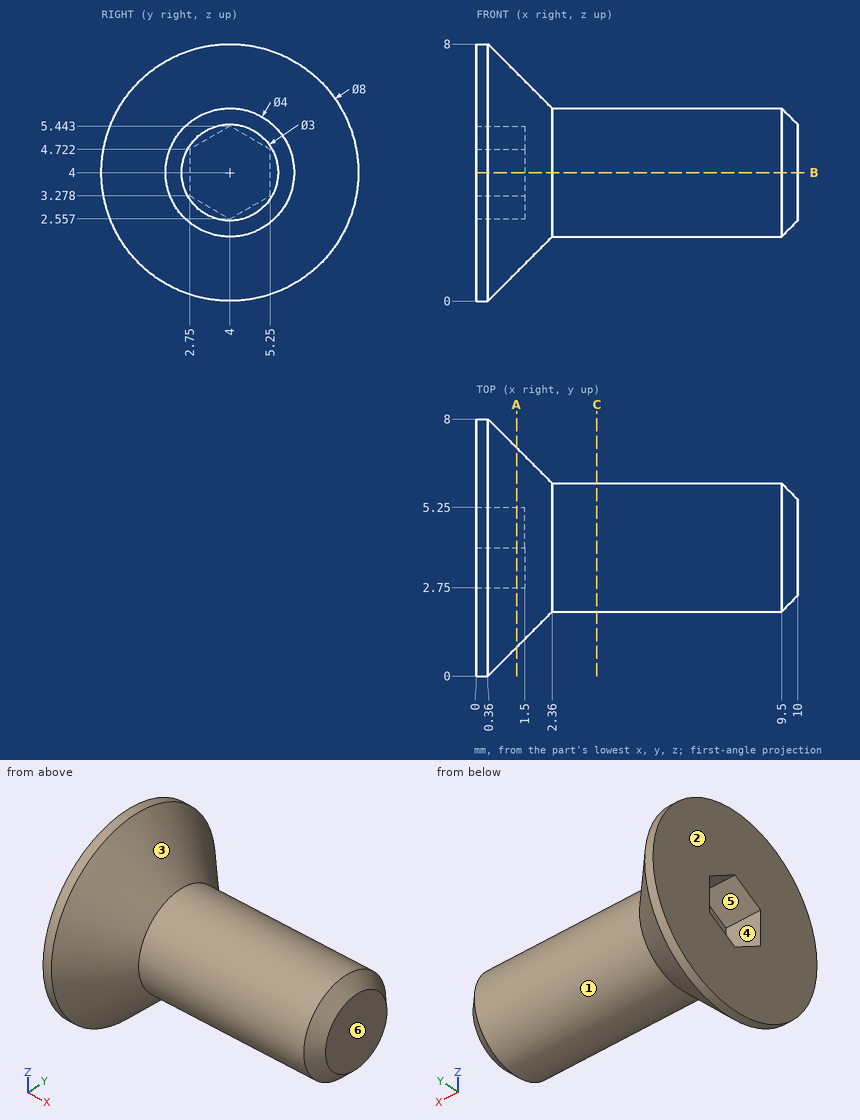
Source: three-view drawing plus pictorial views. Frame: mm from the lowest corner of the part. A direction names the side the tool comes from. Round coordinates to 2 decimals unless told otherwise and drop trailing zeros. Loops run counter-clockwise (first coordinate to the right, second up) from the corner with the lowest first, then second, coordinate; pieces in that order, holes last.
Item 1: Section B-B, the plane z = 4. Output: boundary loops of the cut face in (x, y).
Checked values:
outline: (0, 0) - (0.36, 0) - (2.36, 2) - (9.5, 2) - (10, 2.5) - (10, 5.5) - (9.5, 6) - (2.36, 6) - (0.36, 8) - (0, 8) - (0, 5.25) - (1.5, 5.25) - (1.5, 2.75) - (0, 2.75) - close
Item 2: Section A-A, the plane x = 1.25. Output: boundary loops of the cut face in (y, z).
Checked values:
outline: circle Ø6.22 at (4, 4); hole (2.75, 3.28) - (4, 2.56) - (5.25, 3.28) - (5.25, 4.72) - (4, 5.44) - (2.75, 4.72) - close
Item 3: Mould query, pull axis Y, two halves, no side actions, for the marked faces 3, 4, 5 and 6. Classes: released by +Y, released by -Y, zero draft, split by the parting line, or undercut.
Checked values:
face 3: split by the parting line
face 4: undercut
face 5: undercut
face 6: zero draft
Item 4: Reachability of the marked faces 1 and 2 from +Z, -Z, +X, -X, +Y, -Y: full face, straight path, thin tool, end or side. Return the list, or none.
Checked values:
face 1: +X
face 2: +Z, -Z, -X, +Y, -Y
Item 5: Section C-C, the plane x = 3.75. Output: boundary loops of the cut face in (y, z), plus the area to 3 significant figures.
Checked values:
outline: circle Ø4 at (4, 4)
area: 12.6 mm2
Item 6: Contact query for flat-ended pins moving along their axis: P1, Ø4, axis at x = 7, y = 6, coming from the -Z side; P2, Ø3, axis at x = 9, z = 3.5, coming from the +Y side; P3, Ø3, axis at x = 2, z = 2.5, coming from the +Y side (1 decimal). Output: stop coordinate, or through.
Checked values:
P1: stops at z = 2
P2: stops at y = 6
P3: stops at y = 7.6
Item 7: Line query: L1, parallel to X at y = 4.5, z = 4.75; L2, parallel to Y at x = 1, z = 3.75; L3, parallel to Z at x = 9.25, y = 4. Output: solid intervals per line, ascending.
Checked values:
L1: x = 1.5 to 10
L2: y = 0.65 to 2.75, 5.25 to 7.35
L3: z = 2 to 6
